Geometry: see drawing. Coordinates: mm, zero at the bounding-box minimum. A direction names the side the tool comes from. Round coordinates to 2 decimals unless told otherwise and drop trailing zeros. Loops run counter-clockwise (first coordinate to the right, second up) from the corner with the lowest first, then second, coordinate; pieces in that order, holes last. Notation, with made-up numbers: (-39, 68) -> (-2, 68) arc R11 ccw to (-2, 74) -> close; hole circle Ø1 at (21, -28.75). An arc over 180 degrees is marked (long way). Answer in a Markdown table with one row per item.
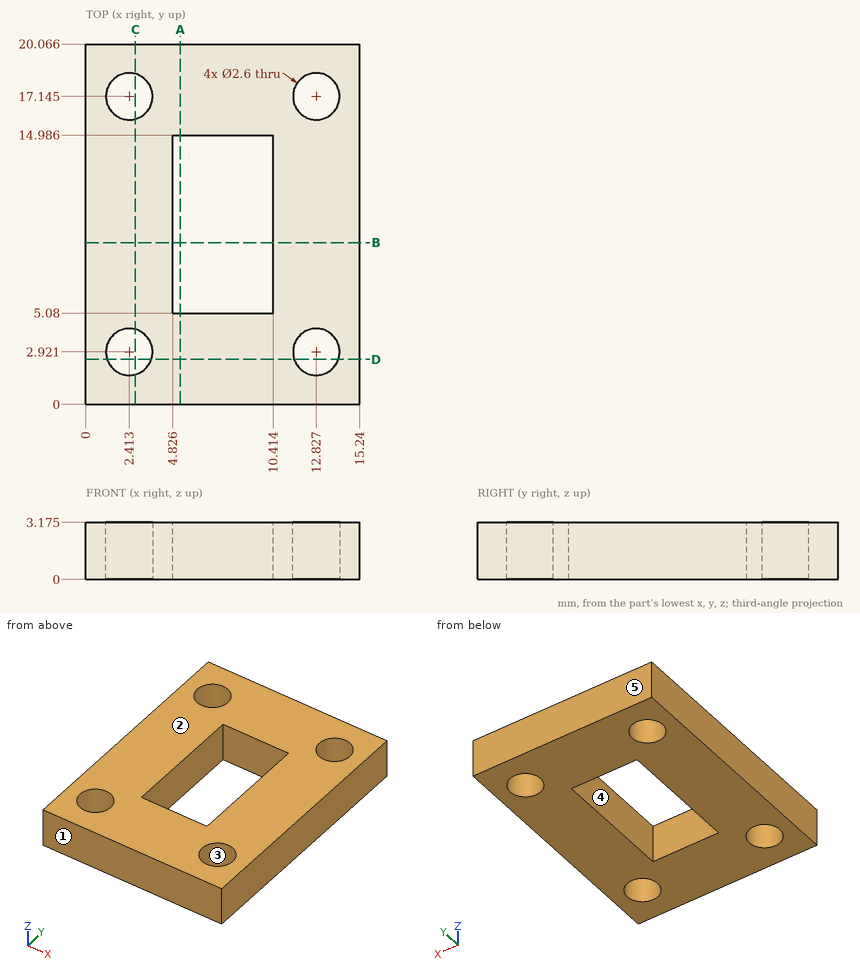
Item 1: Set-up query: the marked faces 4 and 5. Return all of +Z, -Z, +X, -X, +Y, -Y with unobstructed straight access to the full face (end or side cutting, diameter ignored); none if empty.
Ans:
| item | result |
|---|---|
| face 4 | +Z, -Z |
| face 5 | +Z, -Z, +X, -X, +Y |
Item 2: Ray query, L1, parallel to X at y = 14.5, z = 2.15; L2, parallel to Y at x = 12.75, z = 0.95; L3, parallel to X at y = 3.5, z = 1.2. Return the intervals inside material, ascending.
Ans:
| item | result |
|---|---|
| L1 | 0 to 4.83, 10.41 to 15.24 |
| L2 | 0 to 1.62, 4.22 to 15.85, 18.44 to 20.07 |
| L3 | 0 to 1.25, 3.58 to 11.66, 13.99 to 15.24 |
Item 3: Section query D-D, the plane y = 2.5. Output: boundary loops of the cut face in (x, z) (3 decimals).
Ans:
| item | result |
|---|---|
| outline | (0, 0) -> (1.183, 0) -> (1.183, 3.175) -> (0, 3.175) -> close; (3.643, 0) -> (11.597, 0) -> (11.597, 3.175) -> (3.643, 3.175) -> close; (14.057, 0) -> (15.24, 0) -> (15.24, 3.175) -> (14.057, 3.175) -> close |
Item 4: Section query B-B, the plane y = 9. Output: boundary loops of the cut face in (x, z) (3 decimals), and give its area (3 significant figures).
Ans:
| item | result |
|---|---|
| outline | (0, 0) -> (4.826, 0) -> (4.826, 3.175) -> (0, 3.175) -> close; (10.414, 0) -> (15.24, 0) -> (15.24, 3.175) -> (10.414, 3.175) -> close |
| area | 30.6 mm2 |
Item 5: Mould query, pull axis Y, two halves, no side actions, for the marked faces 1, 2 and 3. Classes: released by +Y, released by -Y, zero draft, split by the parting line, or undercut.
Ans:
| item | result |
|---|---|
| face 1 | released by -Y |
| face 2 | zero draft |
| face 3 | undercut |
Item 6: Section query A-A, the plane x = 5.25. Output: boundary loops of the cut face in (y, z) (3 decimals).
Ans:
| item | result |
|---|---|
| outline | (0, 0) -> (5.08, 0) -> (5.08, 3.175) -> (0, 3.175) -> close; (14.986, 0) -> (20.066, 0) -> (20.066, 3.175) -> (14.986, 3.175) -> close |
Item 7: Section query C-C, the plane x = 2.75. Output: boundary loops of the cut face in (y, z) (3 decimals), and give its area (3 significant figures).
Ans:
| item | result |
|---|---|
| outline | (0, 0) -> (1.665, 0) -> (1.665, 3.175) -> (0, 3.175) -> close; (4.177, 0) -> (15.889, 0) -> (15.889, 3.175) -> (4.177, 3.175) -> close; (18.401, 0) -> (20.066, 0) -> (20.066, 3.175) -> (18.401, 3.175) -> close |
| area | 47.8 mm2 |
